```python
from build123d import *

# Parameters (mm, degrees)
BOSS_EXTRUDE1_DEPTH = 550
BOSS_EXTRUDE2_DEPTH = 10


with BuildPart() as part:
    # Sketch1 → Boss-Extrude1 (new body)
    with BuildSketch(Plane(origin=(0, 0, 0), x_dir=(1, 0, 0), z_dir=(0, 1, 0))):
        Polygon((-25, 25), (-5, 25), (-5, 12.5), (5, 12.5), (5, 25), (25, 25), (25, 5), (12.5, 5), (12.5, -5), (25, -5), (25, -25), (5, -25), (5, -12.5), (-5, -12.5), (-5, -25), (-25, -25), (-25, -5), (-12.5, -5), (-12.5, 5), (-25, 5), align=None)
    extrude(amount=BOSS_EXTRUDE1_DEPTH)

    # Sketch1<2> → Boss-Extrude2 (add)
    with BuildSketch(Plane(origin=(0, 0, 0), x_dir=(1, 0, 0), z_dir=(0, 1, 0))):
        Polygon((-25, 25), (-5, 25), (-5, 12.5), (5, 12.5), (5, 25), (25, 25), (25, 5), (12.5, 5), (12.5, -5), (25, -5), (25, -25), (5, -25), (5, -12.5), (-5, -12.5), (-5, -25), (-25, -25), (-25, -5), (-12.5, -5), (-12.5, 5), (-25, 5), align=None)
    extrude(amount=BOSS_EXTRUDE2_DEPTH)


solid = part.part
```
Geometry: final body of the model. Coordinates: model frame, mm. A direction names the side the tool comes from. Coordinates: 2 decimals unless noted, no trailing zeros. Order: outer loops, then holes, each group sorted by start corner. A loop starts at its lowest first (then second) coordinate and runs counter-clockwise, first axis right, second up. Notation, with made-up numbers: (56.5, 70) - (87.5, 70) arc R24 ccw to (87.5, 83) - close; hole circle Ø7 at (22, 62). An arc over 180 degrees is marked (long way). Return JSON: item names as keys, results as strings. Group by question number.
1. Pull-direction query (Z, two-part tool) for faces 5 (the face through (-5, 271, -19)), 6 (the face through (19, 271, -5)), 7 (the face through (-15, 271, 25)); classes: pulls with the +Z half, pulls with the -Z half, needs draft (parallel to the pull), parting line crosses it, or undercut.
2. Material intervals for line 1 along Z through (x, y) = (22.5, 420); line 2 along X through (y, z) = (100, 0), sorted ascending. Write a range as [from, to].
3. Cut plane B-B (x = -17.5). Output: boundary loops of the cut face in (y, z), plus the area to 3 significant figures.
4. Set-up query: faces 1 (the face through (12.5, 271, 0)), 2 (the face through (0, 271, -12.5)), 3 (the face through (0, 271, 12.5)), 4 (the face through (-12.5, 271, 0)). Return all of +Z, -Z, +X, -X, +Y, -Y with unobstructed straight access to the full face (end or side cutting, diameter ignored); none if empty.
5. Cut plane C-C (y = 55). Output: boundary loops of the cut face in (x, z).
6. Cut plane A-A (z = 17). Output: boundary loops of the cut face in (x, y).
7. Pin query (flat end, axial travel): pin 1 (4 mm diameter, centred on x = 0.5, z = 2.5, fed in from -Y); pin 2 (5 mm diameter, centred on y = 161, z = 1.5, fed in from -X); pin 3 (5 mm diameter, centred on x = -1, y = 166.5, fed in from +Z). Return the tip coordinate at first contact, or that it passes through.
Resolved:
{
 "1": {"face 5": "needs draft", "face 6": "undercut", "face 7": "pulls with the +Z half"},
 "2": {"line 1": "z = [-25, -5], [5, 25]", "line 2": "x = [-12.5, 12.5]"},
 "3": {"outline": "(0, -25) - (550, -25) - (550, -5) - (0, -5) - close; (0, 5) - (550, 5) - (550, 25) - (0, 25) - close", "area": "22,000 mm²"},
 "4": {"face 1": "+X, +Y, -Y", "face 2": "-Z, +Y, -Y", "face 3": "+Z, +Y, -Y", "face 4": "-X, +Y, -Y"},
 "5": {"outline": "(-25, -25) - (-5, -25) - (-5, -12.5) - (5, -12.5) - (5, -25) - (25, -25) - (25, -5) - (12.5, -5) - (12.5, 5) - (25, 5) - (25, 25) - (5, 25) - (5, 12.5) - (-5, 12.5) - (-5, 25) - (-25, 25) - (-25, 5) - (-12.5, 5) - (-12.5, -5) - (-25, -5) - close"},
 "6": {"outline": "(-25, 0) - (-5, 0) - (-5, 550) - (-25, 550) - close; (5, 0) - (25, 0) - (25, 550) - (5, 550) - close"},
 "7": {"pin 1": "stops at y = 0", "pin 2": "stops at x = -12.5", "pin 3": "stops at z = 12.5"}
}
